Geometry: final body of the model. Coordinates: model frame, mm. A direction names the side the tool comes from. Give positions to 0.01 mm unless a question says otherwise; leave off trailing zeros. Write each loop counter-clockwise with the first axis right and the second up, starting at its lowest first coordinate (ties: lowest second). Pieces come first, ordered by that corner, then holes. Notation, with made-up numbers: M 82,-28.75 L 93,-28.75 A16 cw 93,-24.75 Z; hole C 29.5,62 d5. An arc over 180 degrees is marked long. One line per question, with ' | ' between items.
from build123d import *

# Parameters (mm, degrees)
SKETCH1_W      = 90
SKETCH1_H      = 60
EXTRUDE1_DEPTH = 50
EXTRUDE2_DEPTH = 91
EXTRUDE3_DEPTH = 75


with BuildPart() as part:
    # Sketch1 → Extrude1 (new body)
    with BuildSketch(Plane(origin=(0, 0, 0), x_dir=(1, 0, 0), z_dir=(0, 1, 0))):
        with Locations((45, 30)):
            Rectangle(SKETCH1_W, SKETCH1_H)
    extrude(amount=EXTRUDE1_DEPTH)

    # Sketch2 → Extrude2 (cut, through all)
    with BuildSketch(Plane(origin=(90, 0, 0), x_dir=(0, 0, -1), z_dir=(1, 0, 0))):
        Polygon((0, 0), (28.867513459, 50), (0, 50), align=None)
    extrude(amount=-EXTRUDE2_DEPTH, mode=Mode.SUBTRACT)

    # Sketch3 → Extrude3 (add)
    with BuildSketch(Plane(origin=(0, 0, 0), x_dir=(1, 0, 0), z_dir=(0, 1, 0))):
        Polygon((90, 60), (90, 0), (75, 0), (45, 60), align=None)
    extrude(amount=EXTRUDE3_DEPTH)


solid = part.part
(1) Cut plane A-A, the plane z = -42. Return loops of the section in (x, y), then the cut area to 3 significant figures.
Working result:
outline: M 0,0 L 90,0 L 90,75 L 54,75 L 54,50 L 0,50 Z | area: 5,400 mm^2
(2) Cut plane B-B, the plane x = 56. Return loops of the section in (y, z).
Working result:
outline: M 0,-60 L 75,-60 L 75,-38 L 50,-38 L 50,-28.87 L 0,0 Z
(3) Set-up query: faces 4 (the face through (44, 29, -60)), 5 (the face through (63.543, 53.642, -22.913)). Return all of +Z, -Z, +X, -X, +Y, -Y with unobstructed straight access to the full face (end or side cutting, diameter ignored); none if empty.
Working result:
face 4: -Z, +X, -X, +Y, -Y | face 5: +Z, -X, +Y
(4) Material intervals for L1, parallel to Y at x = 17, z = -41.5; L2, parallel to X at y = 39.5, z = -17; L3, parallel to Z at x = 19.5, y = 16.5, sorted ascending. Write a range as [from, to].
Working result:
L1: y = [0, 50] | L2: x = [66.5, 90] | L3: z = [-60, -9.53]
(5) Cut plane C-C, the plane x = 33. Return loops of the section in (y, z), then the cut area to 3 significant figures.
Working result:
outline: M 0,-60 L 50,-60 L 50,-28.87 L 0,0 Z | area: 2,280 mm^2
(6) Draft query along Y for faces 1 (the face through (44, 0, -30)), 2 (the face through (83, 37, 0)), 3 (the face through (73, 75, -37)). Return one class per face: released by +Y, released by -Y, zero draft, split by the parting line, or undercut.
Working result:
face 1: released by -Y | face 2: zero draft | face 3: released by +Y
(7) First-contact query: P1, Ø2, axis at y = 62, z = -27, coming from the -X side; P2, Ø3, axis at x = 60, z = -8, coming from the +Y side; P3, Ø1.5, axis at x = 70, y = 26, coming from the +Z side. Flat tips, straight axial feed; report the tip coordinate or a pass-through.
Working result:
P1: stops at x = 61 | P2: stops at y = 16.45 | P3: stops at z = -8.5
(8) Cut plane D-D, the plane x = 66. Return loops of the section in (y, z).
Working result:
outline: M 0,-60 L 75,-60 L 75,-18 L 31.18,-18 L 0,0 Z
